Build history of the part. All positions in model axes, mm. Face numbers are marked on the shaded views. A direction names the side the tool comes from. Round coordinates to 2 decimals unless told otherwise and drop trailing zeros. Loops run counter-clockwise (first coordinate to the right, second up) from the corner with the lowest first, then second, coordinate; pieces in that order, holes last. Notation, with made-up numbers: (-39, 63.5) -> (4, 63.5) arc R32 ccw to (4, 101.5) -> close; hole circle Ø1 at (81.5, 15). An arc over 180 degrees is marked (long way). Put each result on its own line as item: value. Start each with the question number.
Item 1: Tool access for the marked faces 1, 2, 3, 4 and 5: list every direction of +Z, -Z, +X, -X, +Y, -Y with a clear straight run to the whole face (end or side of a thin tool).
Item 2: Cut at D-D, the plane y = 18. List the corners of the cut face in (x, z).
Item 3: Flat gauge pins, fed straight in: pin 1 Ø4 at (x, z) = (-11, 5.5) entering from -Y; pin 2 Ø5 at (x, z) = (-20, 12) entering from -Y; pin 3 Ø5 at (x, y) = (-8.5, -17) entering from -Z. Where does each tip first touch, or does it go through?
Item 4: Cut at C-C, the plane x = 1.5. List the corners of the cut face in (y, z).
Item 5: Pull direction Y, two halves, no side cores. Call the marked faces 6, 7, 8 and 9: +Y half, -Y half, draft (parallel to the pull), parting line (faces both ways), or undercut.
Item 6: Cut at A-A, the plane y = 0. List the corners of the cut face in (x, z) (3 decimals), plus the area to 3 significant figures.
Item 7: Cut at B-B, the plane z = -9.5. List the corners of the cut face in (x, y) (3 decimals), plus the area to 3 significant figures.
Item 8: Drill centre lines: probe 1 along X at (y, z) = (0, 11) (3 decimals); probe 2 along X at (y, z) = (0, -17). Where is each one in solid material? Low to high. Write a range as [from, to].
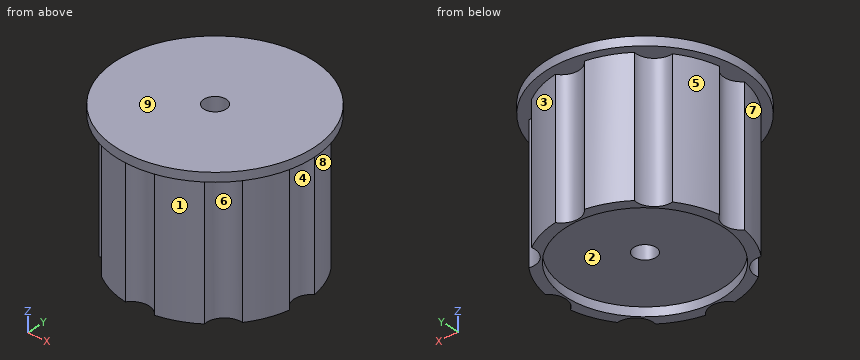
```python
from build123d import *

# Parameters (mm, degrees)
F0_R            = 25.4
F1_DEPTH        = 19.05
F2_R            = 27.94
F2_R_2          = 25.4
F3_DEPTH        = 2.54
F4_R            = 22.352
F5_DEPTH        = 2.54
F6_R            = 3.175
F7_DEPTH        = 38.101
F9_DEPTH        = 38.1
F9_COPIES_COUNT = 8


# Not quite as in the source:
# - a pattern or mirror of a feature is missing from the dataset's text; its kind, count and spacing are read off the source's solid


with BuildPart() as f1:
    # F0 (on Top) → F1 (new body, symmetric)
    with BuildSketch(Plane.XY):
        Circle(F0_R)
    extrude(amount=F1_DEPTH, both=True)

    # F2 (on face) → F3 (join)
    with BuildSketch(Plane.XY.offset(19.05)):
        Circle(F2_R)
        Circle(F2_R_2, mode=Mode.SUBTRACT)
        Circle(F2_R_2)
    extrude(amount=F3_DEPTH)

    # F4 (on face) → F5 (cut)
    with BuildSketch(Plane(origin=(0, 0, -19.05), x_dir=(1, 0, 0), z_dir=(0, 0, -1))):
        Circle(F4_R)
    extrude(amount=-F5_DEPTH, mode=Mode.SUBTRACT)

    # F6 (on face) → F7 (cut, through all)
    with BuildSketch(Plane(origin=(0, 0, -16.51), x_dir=(1, 0, 0), z_dir=(0, 0, -1))):
        Circle(F6_R)
    extrude(amount=-F7_DEPTH, mode=Mode.SUBTRACT)

    # F8 (on face) → F9 (cut, through all)
    with BuildSketch(Plane(origin=(0, 0, -19.05), x_dir=(1, 0, 0), z_dir=(0, 0, -1))):
        with BuildLine():
            ThreePointArc((4.1803474687, 25.0536363636), (0, 25.4), (-4.1803474687, 25.0536363636))
            ThreePointArc((-4.1803474687, 25.0536363636), (0, 22.86), (4.1803474687, 25.0536363636))
        make_face()
    f9 = extrude(amount=-F9_DEPTH, mode=Mode.SUBTRACT)

    # F9_copies: F9 ×8 about axis
    f9_copies_axis = Axis((0, 0, 0), (0, 0, 1))
    for i in range(1, F9_COPIES_COUNT):
        add(f9.rotate(f9_copies_axis, i * 360 / F9_COPIES_COUNT), mode=Mode.SUBTRACT)


solid = f1.part
```
Reply:
1. face 1: -Z, +X, -Y
1. face 2: -Z
1. face 3: -Z, +X, +Y
1. face 4: -Z, +X
1. face 5: -Z, -X, +Y
2. outline: (-21.37, 19.05) -> (-14.99, 19.05) -> (-14.99, -19.05) -> (-13.25, -19.05) -> (-13.25, -16.51) -> (13.25, -16.51) -> (13.25, -19.05) -> (14.99, -19.05) -> (14.99, 19.05) -> (21.37, 19.05) -> (21.37, 21.59) -> (-21.37, 21.59) -> close
3. pin 1: stops at y = -23.75
3. pin 2: stops at y = -15.21
3. pin 3: stops at z = -16.51
4. outline: (-27.9, 19.05) -> (-23.09, 19.05) -> (-23.09, -19.05) -> (-22.3, -19.05) -> (-22.3, -16.51) -> (-2.8, -16.51) -> (-2.8, 21.59) -> (-27.9, 21.59) -> close; (2.8, -16.51) -> (22.3, -16.51) -> (22.3, -19.05) -> (23.09, -19.05) -> (23.09, 19.05) -> (27.9, 19.05) -> (27.9, 21.59) -> (2.8, 21.59) -> close
5. face 6: undercut
5. face 7: -Y half
5. face 8: +Y half
5. face 9: draft
6. outline: (-27.94, 19.05) -> (-22.86, 19.05) -> (-22.86, -19.05) -> (-22.352, -19.05) -> (-22.352, -16.51) -> (-3.175, -16.51) -> (-3.175, 21.59) -> (-27.94, 21.59) -> close; (3.175, -16.51) -> (22.352, -16.51) -> (22.352, -19.05) -> (22.86, -19.05) -> (22.86, 19.05) -> (27.94, 19.05) -> (27.94, 21.59) -> (3.175, 21.59) -> close
6. area: 1,530 mm^2
7. outline: (-25.054, -4.18) arc R25.4 ccw to (-20.672, -14.76) arc R5.08 cw to (-14.76, -20.672) arc R25.4 ccw to (-4.18, -25.054) arc R5.08 cw to (4.18, -25.054) arc R25.4 ccw to (14.76, -20.672) arc R5.08 cw to (20.672, -14.76) arc R25.4 ccw to (25.054, -4.18) arc R5.08 cw to (25.054, 4.18) arc R25.4 ccw to (20.672, 14.76) arc R5.08 cw to (14.76, 20.672) arc R25.4 ccw to (4.18, 25.054) arc R5.08 cw to (-4.18, 25.054) arc R25.4 ccw to (-14.76, 20.672) arc R5.08 cw to (-20.672, 14.76) arc R25.4 ccw to (-25.054, 4.18) arc R5.08 cw to start; hole circle Ø6.35 at (0, 0)
7. area: 1,880 mm^2
8. probe 1: x = [-22.86, -3.175], [3.175, 22.86]
8. probe 2: x = [-22.86, -22.35], [22.35, 22.86]
